Source: CAD feature listing. Evaluate the final solid. Frame: model axes, mm. Give positions to 0.01 mm unless a question says otherwise; leave off trailing zeros. Order: outer loops, then holes, each group sorted by start corner. A loop starts at its lowest first (then second) coordinate and runs counter-clockwise, first axis right, second up. Notation, with made-up numbers: (76.5, 17.5) - (92.5, 17.5) arc R34 cw to (92.5, 56.5) - close; hole circle Ø7 at (50, 68). An arc over 180 degrees is marked (long way). Answer as CSV lines item,"result".
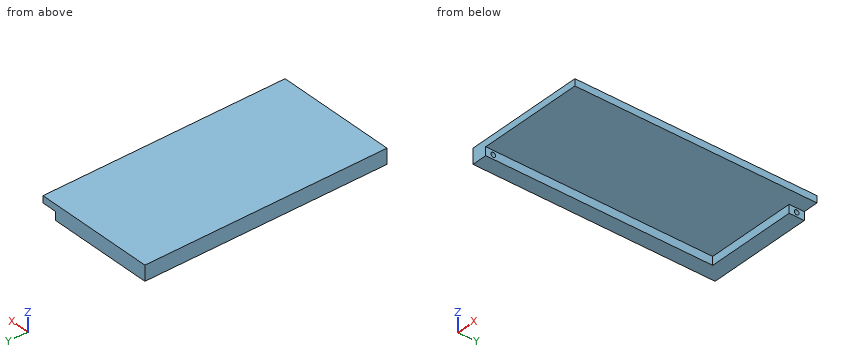
```python
from build123d import *

# Parameters (mm, degrees)
F0_W     = 25.4
F0_H     = 25.4
F0_H_2   = 381
F0_W_2   = 152.4
F1_DEPTH = 25.4
F2_DEPTH = 11.43
F4_R     = 3.96875
F5_DEPTH = 12.7
F3_R     = 3.96875
F6_DEPTH = 12.7


with BuildPart() as f1:
    # F0 (on Top) → F1 (new body)
    with BuildSketch(Plane.XY):
        with Locations((-88.9, 190.5)):
            Rectangle(F0_W, F0_H)
        with Locations((-88.9, -12.7)):
            Rectangle(F0_W, F0_H_2)
        with Locations((0, 190.5)):
            Rectangle(F0_W_2, F0_H)
    extrude(amount=-F1_DEPTH)

    # F0 (on Top) → F2 (join)
    with BuildSketch(Plane.XY):
        with Locations((-88.9, 190.5)):
            Rectangle(F0_W, F0_H)
        with Locations((-88.9, -12.7)):
            Rectangle(F0_W, F0_H_2)
        with Locations((0, 190.5)):
            Rectangle(F0_W_2, F0_H)
        Polygon((101.6, -203.2), (101.6, 177.8), (76.2, 177.8), (-76.2, 177.8), (-76.2, -203.2), align=None)
        with Locations((88.9, 190.5)):
            Rectangle(F0_W, F0_H)
    extrude(amount=-F2_DEPTH)

    # F4 (on face) → F5 (cut)
    with BuildSketch(Plane.YZ.offset(76.2)):
        with Locations((190.5, -18.415)):
            Circle(F4_R)
    extrude(amount=-F5_DEPTH, mode=Mode.SUBTRACT)

    # F3 (on face) → F6 (cut)
    with BuildSketch(Plane.YZ.offset(-76.2)):
        with Locations((-190.5, -18.415)):
            Circle(F3_R)
    extrude(amount=-F6_DEPTH, mode=Mode.SUBTRACT)


solid = f1.part
```
(1) Cut plane D-D (x = 89). Return loops of the section in (y, z).
Completed:
outline,"(-203.2, -11.43) - (203.2, -11.43) - (203.2, 0) - (-203.2, 0) - close"
(2) Ray query, line 1 (Z direction, x = 71.75, y = 190.5); line 2 (X direction, y = 65, z = -20.5); line 3 (Z direction, x = -71, y = 68). Return the intervals inside material, ascending. Write a range as from..to.
Completed:
line 1,"-25.4..-22.38, -14.45..0"
line 2,"-101.6..-76.2"
line 3,"-11.43..0"
(3) Cut plane C-C (y = -190.5). Return loops of the section in (x, z).
Completed:
outline,"(-101.6, -25.4) - (-76.2, -25.4) - (-76.2, -22.38) - (-88.9, -22.38) - (-88.9, -14.45) - (-76.2, -14.45) - (-76.2, -11.43) - (101.6, -11.43) - (101.6, 0) - (-101.6, 0) - close"
(4) Cut plane B-B (x = -15). Return loops of the section in (y, z).
Completed:
outline,"(-203.2, -11.43) - (177.8, -11.43) - (177.8, -25.4) - (203.2, -25.4) - (203.2, 0) - (-203.2, 0) - close"
(5) Contact query for flat-ended pins moving along their axis: pin 1 (3 mm diameter, centred on x = 26, z = -13, fed in from -Y); pin 2 (4 mm diameter, centred on y = 190, z = -20, fed in from +X); pin 3 (3 mm diameter, centred on y = 116.5, z = -16, fed in from +X). Output: stop coordinate, or through.
Completed:
pin 1,"y = 177.8"
pin 2,"x = 63.5"
pin 3,"x = -76.2"
(6) Cut plane A-A (y = 190.5). Return loops of the section in (x, z).
Completed:
outline,"(-101.6, -25.4) - (76.2, -25.4) - (76.2, -22.38) - (63.5, -22.38) - (63.5, -14.45) - (76.2, -14.45) - (76.2, -11.43) - (101.6, -11.43) - (101.6, 0) - (-101.6, 0) - close"
